```python
from build123d import *

# Parameters (mm, degrees)
F0_W     = 150
F0_H     = 140
F1_DEPTH = 85
F2_R     = 2.765875
F3_DEPTH = 10


with BuildPart() as f1:
    # F0 (on Front) → F1 (new body)
    with BuildSketch(Plane.XZ):
        with Locations((1.931816, -3.698107)):
            Rectangle(F0_W, F0_H)
    extrude(amount=F1_DEPTH)

    # F2 (on face) → F3 (cut)
    with BuildSketch(Plane.XY.offset(66.301893)):
        with Locations((-67.068184, -5)):
            Circle(F2_R)
        with Locations((-67.068184, -69)):
            Circle(F2_R)
        with Locations((70.931816, -5)):
            Circle(F2_R)
        with Locations((46.931816, -79)):
            Circle(F2_R)
    extrude(amount=-F3_DEPTH, mode=Mode.SUBTRACT)


solid = f1.part
```
Could you check a few things on this model? Use its own coordinates, in mm. A direction names the side the tool comes from. Coordinates: 2 decimals unless noted, no trailing zeros. One line per question, with ' | ' between items. Start each with the question number.
1. Thinking about a two-plate mould opening in X: for faces 1 (the face through (76.932, -42, -5)), 2 (the face through (71, -5, 56.302)), 3 (the face through (1, -42, 66.302)), which applies, pulls with the +X half, pulls with the -X half, needs draft (parallel to the pull), parting line crosses it, or undercut?
2. For faces 4 (the face through (68.17, -4.88, 61.37)), 5 (the face through (-73.068, -42, -5)), which set-ups out of +Z, -Z, +X, -X, +Y, -Y let a thin tool reach every point of the face, with its end or its side?
3. Will this pin go through, and if not, where does the flat tip stop? P1, Ø5, axis at x = 46.93, y = -79, coming from the +Z side.
Return value:
1) face 1: pulls with the +X half | face 2: undercut | face 3: needs draft
2) face 4: +Z | face 5: +Z, -Z, -X, +Y, -Y
3) P1: stops at z = 56.3
